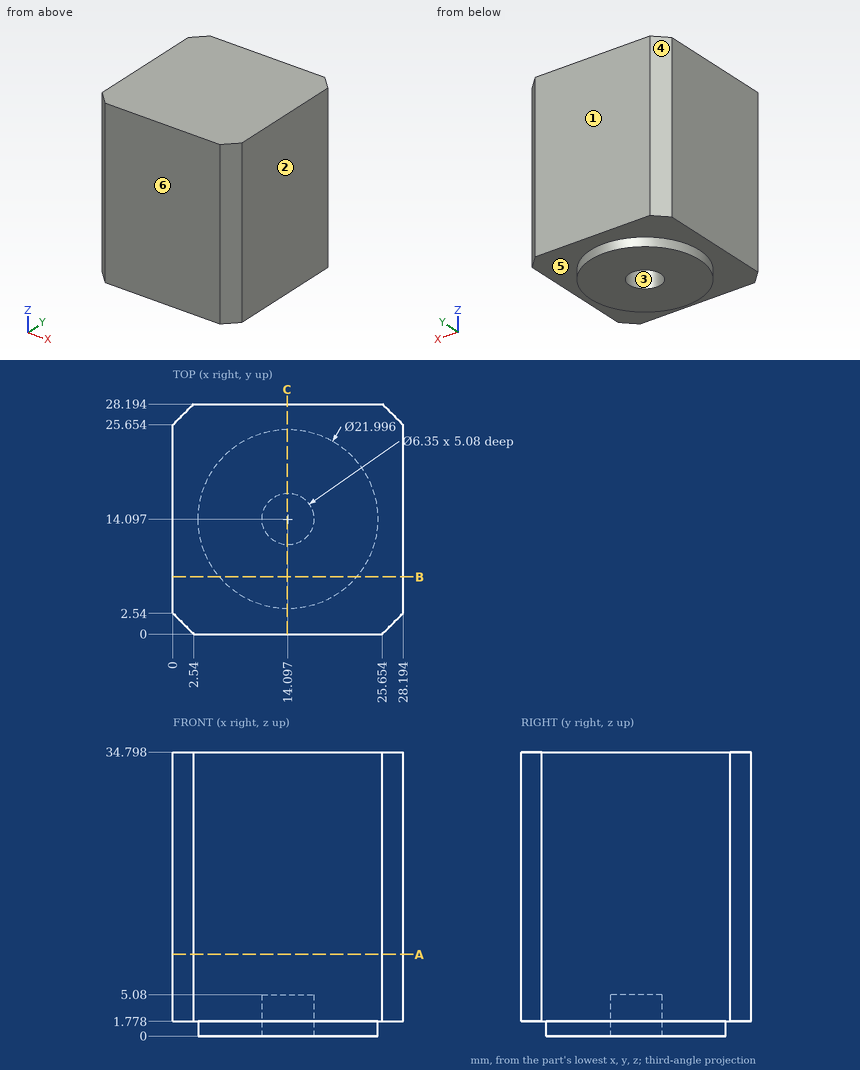
Verification items for this drawing (mm, ordinates from the low corner). A direction names the side the tool comes from. Give positions to 0.01 mm unless a question says otherwise; leave off trailing zeros. Loops run counter-clockwise (first coordinate to the right, second up) from the corner with the lowest first, then second, coordinate; pieces in that order, holes last. Notation, with made-up numbers: M -16.75,85 L -6.75,85 A28 cw -6.75,115 Z; hole C -18.5,34.5 d1. An arc over 180 degrees is marked long. Answer as a JSON object with one key per item and string values. Group by question number.
Q1. Cross-section at B-B on y = 7. Record the cut outline in (x, z) (1 decimal).
Q2. Release check for a two-part mould opening along X. For the marked faces 1, 2, 3 and 4 record: released by +X, released by -X, zero draft, split by the parting line, or undercut.
Q3. Access from +Z, -Z, +X, -X, +Y, -Y to the whole of each face (thin tool, end or side, straight path). Record for the marked faces 5 and 6.
Q4. Material ranges on line 1 along Z through (x, y) = (25.75, 23); line 2 along Y through (x, z) = (1.75, 28) (1 decimal), recorded low to high. Write a range as [from, to].
Q5. Go/stop test with a flat-tipped pin: P1, Ø5, axis at x = 14.097, y = 14.097, coming from the -Z side. Record where the tip stops, or that it passes through.
Q6. Cross-section at A-A on z = 10. Record the cut outline in (x, y).
Q7. Cross-section at C-C on x = 14. Record the cut outline in (y, z) (1 decimal), then the cut area to 3 significant figures.
Evaluation:
{
 "1": {"outline": "M 0,1.8 L 5.7,1.8 L 5.7,0 L 22.5,0 L 22.5,1.8 L 28.2,1.8 L 28.2,34.8 L 0,34.8 Z"},
 "2": {"face 1": "zero draft", "face 2": "released by +X", "face 3": "undercut", "face 4": "released by -X"},
 "3": {"face 5": "-Z", "face 6": "+Z, -Z, +X, -X, -Y"},
 "4": {"line 1": "z = [1.78, 34.8]", "line 2": "y = [0.8, 27.4]"},
 "5": {"P1": "stops at z = 5.08"},
 "6": {"outline": "M 0,2.54 L 2.54,0 L 25.65,0 L 28.19,2.54 L 28.19,25.65 L 25.65,28.19 L 2.54,28.19 L 0,25.65 Z"},
 "7": {"outline": "M 0,1.8 L 3.1,1.8 L 3.1,0 L 10.9,0 L 10.9,5.1 L 17.3,5.1 L 17.3,0 L 25.1,0 L 25.1,1.8 L 28.2,1.8 L 28.2,34.8 L 0,34.8 Z", "area": "938 mm2"}
}
